from build123d import *

# Parameters (mm, degrees)
F0_W     = 320
F0_H     = 19.95
F0_R     = 2.25
F1_DEPTH = 3
F2_W     = 320
F2_H     = 3
F3_DEPTH = 16.98
F6_R     = 2.25
F7_DEPTH = 3.001


with BuildPart() as f1:
    # F0 (on Top) → F1 (new body)
    with BuildSketch(Plane.XY):
        with Locations((160, 9.975)):
            Rectangle(F0_W, F0_H)
        with Locations((6.05, 9.18)):
            Circle(F0_R, mode=Mode.SUBTRACT)
        with Locations((214.92, 9.18)):
            Circle(F0_R, mode=Mode.SUBTRACT)
        with Locations((282.43, 9.18)):
            Circle(F0_R, mode=Mode.SUBTRACT)
        with Locations((307.4, 9.18)):
            Circle(F0_R, mode=Mode.SUBTRACT)
    extrude(amount=F1_DEPTH)

    # F2 (on face) → F3 (join)
    with BuildSketch(Plane.XY.offset(3)):
        with Locations((160, 18.45)):
            Rectangle(F2_W, F2_H)
    extrude(amount=F3_DEPTH)

    # F6 (on face) → F7 (cut, through all)
    with BuildSketch(Plane.XZ.offset(-16.95)):
        with Locations((307.4, 10.77)):
            Circle(F6_R)
        with Locations((282.43, 10.77)):
            Circle(F6_R)
        with Locations((214.92, 10.77)):
            Circle(F6_R)
        with Locations((6.05, 10.77)):
            Circle(F6_R)
    extrude(amount=-F7_DEPTH, mode=Mode.SUBTRACT)


solid = f1.part
Check sheet for the modelled part. Datum: model origin and axes. Units: mm. A direction names the side the tool comes from. Give positions to 0.01 mm unless a question says otherwise; leave off trailing zeros. Loops run counter-clockwise (first coordinate to the right, second up) from the corner with the lowest first, then second, coordinate; pieces in that order, holes last. Notation, with made-up numbers: M 0.5,38 L 50.5,38 A15 ccw 50.5,49 Z; hole C 69.25,88.5 d10. An arc over 180 degrees is marked long. Return JSON: item names as keys, results as strings. Group by question number.
1. Go/stop test with flat-tipped pins: pin 1 (4 mm diameter, centred on x = 72, y = 8.5, fed in from +Z); pin 2 (5 mm diameter, centred on x = 214.92, z = 10.77, fed in from -Y). Record where each tip stops, or that it passes through.
2. Cross-section at B-B on z = 15.75. Record the boundary of the cut face in (x, y), plus the area to 3 significant figures.
3. Thickness scan on L1, parallel to Y at x = 6.05, z = 1.55; L2, parallel to Z at x = 6.05, y = 18.45; L3, parallel to Y at x = 201.5, z = 7.5. Record the ranges inside material, lowest first.
4. Cross-section at A-A on x = 101.5. Record the boundary of the cut face in (y, z), plus the area to 3 significant figures.
5. Tool access check on faces 1 (the flat face through (158, 10, 0)), 2 (the flat face through (158, 16.95, 11)). Record the directions out of +Z, -Z, +X, -X, +Y, -Y that give a thin tool (end or side, any length) a straight path to the whole face; none if there is none.
Return value:
{
 "1": {"pin 1": "z = 3", "pin 2": "y = 16.95"},
 "2": {"outline": "M 0,16.95 L 320,16.95 L 320,19.95 L 0,19.95 Z", "area": "960 mm^2"},
 "3": {"L1": "0 to 6.93, 11.43 to 19.95", "L2": "0 to 8.52, 13.02 to 19.98", "L3": "16.95 to 19.95"},
 "4": {"outline": "M 0,0 L 19.95,0 L 19.95,19.98 L 16.95,19.98 L 16.95,3 L 0,3 Z", "area": "111 mm^2"},
 "5": {"face 1": "-Z, +X, -X, +Y, -Y", "face 2": "+Z, +X, -X, -Y"}
}
